Autodesk Fusion 360 part; units mm, degrees
sketch "Sketch1" plane through (0, 0, 0) normal (0, 1, 0) x (1, 0, 0)
  circle A0 centre (0, 0) radius 7.2
  circle A1 centre (0, 0) radius 2.55
  line L0 (7.2, 0) -> (2.55, 0)
  line L1 (2.55, 0) -> (2.55, -28.2)
  line L2 (2.55, -28.2) -> (7.2, -28.2)
  line L3 (7.2, -28.2) -> (7.2, 0)
  line L4 (7.2, -28.2) -> (-3.3, -28.2)
  line L5 (-3.3, -28.2) -> (-3.3, -23.55)
  line L6 (-3.3, -23.55) -> (7.2, -23.55)
  line L7 (7.2, -23.55) -> (7.2, -28.2)
  line L8 (2.55, 0) -> (-7.2, 0)
  line L9 (7.2, -5.8) -> (7.2, -1.15)
  line L10 (7.2, -14.1) -> (51.9103, -9.0016)
  line L11 (51.9103, -9.0016) -> (51.3936, -4.471)
  line L12 (51.3936, -4.471) -> (6.6834, -9.5694)
  line L13 (6.6834, -9.5694) -> (7.2, -14.1)
  line L14 (51.9103, -9.0016) -> (47.4463, -7.6995)
  line L15 (47.4463, -7.6995) -> (49.4624, -0.7876)
  line L16 (49.4624, -0.7876) -> (53.9264, -2.0897)
  line L17 (53.9264, -2.0897) -> (51.9103, -9.0016)
  dimension "d1" = 14.4
  dimension "d2" = 5.1
  dimension "d3" = 4.65
  dimension "d4" = 28.2
  dimension "d5" = 10.5
  dimension "d6" = 4.65
  dimension "d16" = 45
  dimension "d17" = 4.56
  dimension "d18" = 4.65
  dimension "d19" = 7.2
extrude "Extrude1" add sketch "Sketch1" along normal blind 4.65 contours A0 A1 L0 L8 | A0 L1 L3 L6 L9 L12 L13 | A0 L0 L1 | L1 L2 L3 L4 L6 L7 | L1 L4 L5 L6 | L3 L10 L12 L14 L15 | L3 L12 L13 | L11 L12 L15 L16 L17 | L11 L12 L14 L15
fillet "Fillet1" radius 2 3 edges at (49.4624, 2.325, 0.7876) (53.9264, 2.325, 2.0897) (51.9103, 2.325, 9.0016)
fillet "Fillet2" radius 2 1 edges at (7.2, 2.325, 28.2)
fillet "Fillet3" radius 2 2 edges at (-0.375, 4.65, 23.55) (-0.375, 0, 23.55)
Verification items for the finished model (mm, model axes). A direction names the side the tool comes from. Give positions to 0.01 mm unless a question says otherwise; leave off trailing zeros. Write each loop counter-clockwise with the first axis right and the second up, starting at its lowest first coordinate (ties: lowest second). Pieces come first, ordered by that corner, then holes. Notation, with made-up numbers: (59, -0.75) - (76, -0.75) arc R25 cw to (76, 11.25) - close; hole circle Ø5 at (-18, 33). An arc over 180 degrees is marked (long way). Put each result on its own line as item: value.
Q1. Section check B-B on y = 3.9. Record the cut outline in (x, z).
Result:
outline: (-7.2, 0) arc R7.2 ccw to (7.2, 0) - (7.2, 9.51) - (48.28, 4.83) - (48.9, 2.71) arc R2 ccw to (51.38, 1.35) - (52.01, 1.53) arc R2 ccw to (53.37, 4.01) - (52.28, 7.73) arc R2 ccw to (50.59, 9.15) - (7.2, 14.1) - (7.2, 26.2) arc R2 ccw to (5.2, 28.2) - (-3.3, 28.2) - (-3.3, 23.99) - (2.55, 23.99) - (2.55, 0) arc R2.55 cw to (-2.55, 0) - close
Q2. Set-up check for faces 1 (the face through (-0.06, 2.29, -2.55)), 2 (the face through (-5, 2, 0)), 3 (the face through (7.2, 2, 5)), 4 (the face through (-0.33, 0.57, 24.15)): record each of +Z, -Z, +X, -X, +Y, -Y from which the full face is reachable in a straight line by a thin tool's end or side.
Result:
face 1: +Y, -Y
face 2: -X, +Y, -Y
face 3: -Z, +Y, -Y
face 4: -X, -Y
Q3. Mould release check, pull along X, two halves, no side actions. Record for faces 5 (the face through (16, 0, 9)), 6 (the face through (28.03, 2.292, 7.135)), 7 (the face through (-3.3, 2, 26)), 8 (the face through (48.59, 2.29, 3.78)): released by +X, released by -X, zero draft, split by the parting line, or undercut.
Result:
face 5: zero draft
face 6: undercut
face 7: released by -X
face 8: undercut
Q4. Section check A-A on x = 0. Record the cut outline in (y, z), and give its area (3 significant figures).
Result:
outline: (0, -7.2) - (4.65, -7.2) - (4.65, -2.55) - (0, -2.55) - close; (0, 25.55) arc R2 ccw to (2, 23.55) - (2.65, 23.55) arc R2 ccw to (4.65, 25.55) - (4.65, 28.2) - (0, 28.2) - close
area: 41.5 mm2
Q5. Scan lines: probe 1 along X at (y, z) = (3.15, 16.5); probe 2 along Z at (x, y) = (-0.5, 3.5); probe 3 along X at (y, z) = (4.1, 4). Record each from-to range of solid material in increasing order. Write a range as from..to.
Result:
probe 1: 2.55..7.2
probe 2: -7.18..-2.5, 23.74..28.2
probe 3: 2.55..7.2, 48.53..53.37
Q6. Section check C-C on z = 18.5. Record the cut outline in (x, y), and give its area (3 significant figures).
Result:
outline: (2.55, 0) - (7.2, 0) - (7.2, 4.65) - (2.55, 4.65) - close
area: 21.6 mm2
Q7. Depth check by flat-ended pin: P1, Ø2, axis at x = 30.5, y = 4, coming from the +Z side; P2, Ø0.7, axis at x = -1.5, y = 2, coming from the -Z side; P3, Ø2.5, axis at y = 3, z = 11, coming from the -X side. Enter the tip coordinate at first touch or a pass-through.
Result:
P1: z = 11.56
P2: z = -7.11
P3: x = 2.55
Q8. Section check D-D on y = 0.65. Record the cut outline in (x, z).
Result:
outline: (-7.2, 0) arc R7.2 ccw to (7.2, 0) - (7.2, 9.51) - (48.28, 4.83) - (48.9, 2.71) arc R2 ccw to (51.38, 1.35) - (52.01, 1.53) arc R2 ccw to (53.37, 4.01) - (52.28, 7.73) arc R2 ccw to (50.59, 9.15) - (7.2, 14.1) - (7.2, 26.2) arc R2 ccw to (5.2, 28.2) - (-3.3, 28.2) - (-3.3, 24.07) - (2.55, 24.07) - (2.55, 0) arc R2.55 cw to (-2.55, 0) - close
